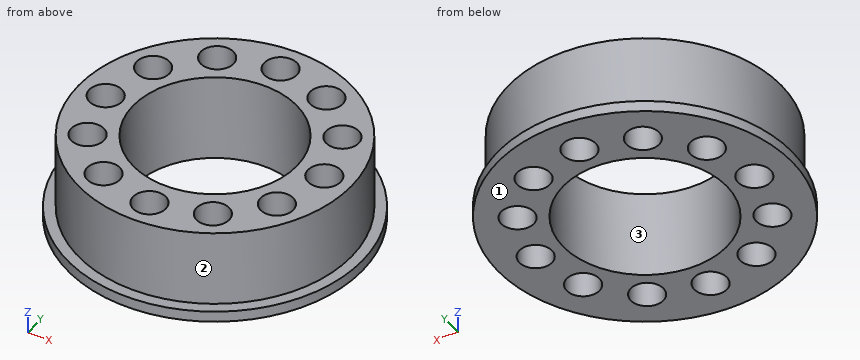
from build123d import *

# Parameters (mm, degrees)
SKETCH_2_R          = 1.5
CUT_EXTRUDE_1_DEPTH = 21.700241544


with BuildPart() as part:
    # ｽｹｯﾁ1 → 回転1 (revolve)
    with BuildSketch(Plane(origin=(0, 0, 0), x_dir=(0, 0, -1), z_dir=(1, 0, 0)), mode=Mode.PRIVATE) as revolve_1_sk:
        Polygon((0, 7.5), (8, 7.5), (8, 13.5), (7, 13.5), (7, 12.5), (0, 12.5), align=None)
    revolve(revolve_1_sk.sketch.rotate(Axis((0, 0, 0), (0, 0, -1)), 90), axis=Axis((0, 0, 0), (0, 0, -1)))

    # ｽｹｯﾁ2 → ｶｯﾄ - 押し出し1 (cut, through all)
    with BuildSketch(Plane.XY):
        with Locations((0, 10)):
            Circle(SKETCH_2_R)
        with Locations((5, 8.660254038)):
            Circle(SKETCH_2_R)
        with Locations((8.660254038, 5)):
            Circle(SKETCH_2_R)
        with Locations((10, 0)):
            Circle(SKETCH_2_R)
        with Locations((8.660254038, -5)):
            Circle(SKETCH_2_R)
        with Locations((5, -8.660254038)):
            Circle(SKETCH_2_R)
        with Locations((0, -10)):
            Circle(SKETCH_2_R)
        with Locations((-5, -8.660254038)):
            Circle(SKETCH_2_R)
        with Locations((-8.660254038, -5)):
            Circle(SKETCH_2_R)
        with Locations((-10, 0)):
            Circle(SKETCH_2_R)
        with Locations((-8.660254038, 5)):
            Circle(SKETCH_2_R)
        with Locations((-5, 8.660254038)):
            Circle(SKETCH_2_R)
    extrude(amount=-CUT_EXTRUDE_1_DEPTH, mode=Mode.SUBTRACT)


solid = part.part
Could you check a few things on this model? Use its own coordinates, in mm. Face numbers are marked on the shaded views. Round coordinates to 2 decimals unless told otherwise and drop trailing zeros. Write each loop counter-clockwise with the first axis right and the second up, starting at its lowest first coordinate (ties: lowest second). Pieces come first, ordered by that corner, then holes. Notation, with made-up numbers: (-8.75, 45) - (44.25, 45) arc R14 ccw to (44.25, 56) - close; hole circle Ø5 at (-19.5, 82.25). An arc over 180 degrees is marked (long way). Put each result on its own line as item: value. Start each with the question number.
(1) I need wall thicknesses on probe 1 along Y at (x, z) = (0, -3.25); probe 2 along Y at (x, z) = (9, -5.75); probe 3 along X at (y, z) = (-0.25, -2). Which ranges of each line are inside material? Lowest first, please.
(2) I want a section at A-A, the plane y = 0. Please give me the cut outline in (x, z).
(3) I want a section at B-B, the plane x = 5. Please give me the cut outline in (y, z).
(4) I want a section at D-D, the plane y = -10.75. Please give me the cut outline in (x, z), plus the area to 3 significant figures.
(5) I want a section at C-C, the plane z = -7.5. Give the number of separate pieces and of enclosed holes in the cut face, plus the area to 3 significant figures.
(6) Will these pins go through, and if not, where does the flat tip stop? pin 1 (1.5 mm diameter, centred on y = -7, z = -2, fed in from +X); pin 2 (2 mm diameter, centred on x = 1, z = -4.5, fed in from -Y); pin 3 (4 mm diameter, centred on y = 2, z = -5.5, fed in from +X).
(7) Thinking about a two-plate mould opening in Y: for the marked faces 1, 2 and 3, which applies, released by +Y, released by -Y, zero draft, split by the parting line, or undercut?
Here are the results:
1. probe 1: y = -12.5 to -11.5, -8.5 to -7.5, 7.5 to 8.5, 11.5 to 12.5
1. probe 2: y = -8.67 to -6.46, -3.54 to -1.12, 1.12 to 3.54, 6.46 to 8.67
1. probe 3: x = -12.5 to -11.48, -8.52 to -7.5, 7.5 to 8.52, 11.48 to 12.5
2. outline: (-13.5, -8) - (-11.5, -8) - (-11.5, 0) - (-12.5, 0) - (-12.5, -7) - (-13.5, -7) - close; (-8.5, -8) - (-7.5, -8) - (-7.5, 0) - (-8.5, 0) - close; (7.5, -8) - (8.5, -8) - (8.5, 0) - (7.5, 0) - close; (11.5, -8) - (13.5, -8) - (13.5, -7) - (12.5, -7) - (12.5, 0) - (11.5, 0) - close
3. outline: (-12.54, -8) - (-10.16, -8) - (-10.16, 0) - (-11.46, 0) - (-11.46, -7) - (-12.54, -7) - close; (-7.16, -8) - (-5.59, -8) - (-5.59, 0) - (-7.16, 0) - close; (5.59, -8) - (7.16, -8) - (7.16, 0) - (5.59, 0) - close; (10.16, -8) - (12.54, -8) - (12.54, -7) - (11.46, -7) - (11.46, 0) - (10.16, 0) - close
4. outline: (-8.17, -8) - (-1.3, -8) - (-1.3, 0) - (-6.38, 0) - (-6.38, -7) - (-8.17, -7) - close; (1.3, -8) - (8.17, -8) - (8.17, -7) - (6.38, -7) - (6.38, 0) - (1.3, 0) - close
4. area: 84.8 mm^2
5. separate pieces: 1
5. enclosed holes: 13
5. area: 311 mm^2
6. pin 1: stops at x = 10.83
6. pin 2: stops at y = -12.5
6. pin 3: stops at x = 13.48
7. face 1: zero draft
7. face 2: split by the parting line
7. face 3: undercut
